```python
from build123d import *

# Parameters (mm, degrees)
F0_R     = 2.4892
F0_R_2   = 2.0193
F0_R_3   = 3.175
F0_R_4   = 1.397
F2_DEPTH = 3
F1_R     = 1.5875
F3_DEPTH = 3.001
F4_W     = 33.02
F4_H     = 15.24
F5_DEPTH = 1.41224


with BuildPart() as f2:
    # F0 (on Top) → F2 (new body)
    with BuildSketch(Plane.XY):
        with BuildLine():
            Line((329.40625, 44.45), (-329.40625, 44.45))
            ThreePointArc((-329.40625, 44.45), (-331.651314, 43.520064), (-332.58125, 41.275))
            Line((-332.58125, 41.275), (-332.58125, -41.275))
            ThreePointArc((-332.58125, -41.275), (-331.651314, -43.520064), (-329.40625, -44.45))
            Line((-329.40625, -44.45), (329.40625, -44.45))
            ThreePointArc((329.40625, -44.45), (331.651314, -43.520064), (332.58125, -41.275))
            Line((332.58125, -41.275), (332.58125, 41.275))
            ThreePointArc((332.58125, 41.275), (331.651314, 43.520064), (329.40625, 44.45))
        make_face()
        with Locations((-326.23125, -38.1)):
            Circle(F0_R, mode=Mode.SUBTRACT)
        with Locations((-121.96875, -35.2)):
            Circle(F0_R_2, mode=Mode.SUBTRACT)
        with Locations((-47.26875, -35.2)):
            Circle(F0_R_2, mode=Mode.SUBTRACT)
        with Locations((-326.23125, -22.225)):
            Circle(F0_R, mode=Mode.SUBTRACT)
        with Locations((-326.23125, -6.35)):
            Circle(F0_R, mode=Mode.SUBTRACT)
        with Locations((27.43125, -35.2)):
            Circle(F0_R_2, mode=Mode.SUBTRACT)
        with Locations((102.13125, -35.2)):
            Circle(F0_R_2, mode=Mode.SUBTRACT)
        with Locations((176.83125, -35.2)):
            Circle(F0_R_2, mode=Mode.SUBTRACT)
        with Locations((251.53125, -35.2)):
            Circle(F0_R_2, mode=Mode.SUBTRACT)
        with Locations((326.23125, -38.1)):
            Circle(F0_R, mode=Mode.SUBTRACT)
        with Locations((326.23125, -22.225)):
            Circle(F0_R, mode=Mode.SUBTRACT)
        with Locations((326.23125, -6.35)):
            Circle(F0_R, mode=Mode.SUBTRACT)
        with Locations((-326.23125, 6.35)):
            Circle(F0_R, mode=Mode.SUBTRACT)
        with Locations((-326.23125, 22.225)):
            Circle(F0_R, mode=Mode.SUBTRACT)
        with Locations((-326.23125, 38.1)):
            Circle(F0_R, mode=Mode.SUBTRACT)
        with Locations((-121.96875, 35.2)):
            Circle(F0_R_2, mode=Mode.SUBTRACT)
        with Locations((-47.26875, 35.2)):
            Circle(F0_R_2, mode=Mode.SUBTRACT)
        with Locations((326.23125, 6.35)):
            Circle(F0_R, mode=Mode.SUBTRACT)
        with Locations((27.43125, 35.2)):
            Circle(F0_R_2, mode=Mode.SUBTRACT)
        with Locations((102.13125, 35.2)):
            Circle(F0_R_2, mode=Mode.SUBTRACT)
        with Locations((326.23125, 22.225)):
            Circle(F0_R, mode=Mode.SUBTRACT)
        with Locations((176.83125, 35.2)):
            Circle(F0_R_2, mode=Mode.SUBTRACT)
        with Locations((251.53125, 35.2)):
            Circle(F0_R_2, mode=Mode.SUBTRACT)
        with Locations((275.43125, 35.2)):
            Circle(F0_R_3, mode=Mode.SUBTRACT)
        with Locations((300.83125, 35.2)):
            Circle(F0_R_4, mode=Mode.SUBTRACT)
        with Locations((326.23125, 38.1)):
            Circle(F0_R, mode=Mode.SUBTRACT)
    extrude(amount=F2_DEPTH)

    # F1 (on face) → F3 (cut, through all)
    with BuildSketch(Plane.XY):
        with BuildLine():
            Line((293.120775, 14.162294), (279.987659, 14.162294))
            ThreePointArc((279.987659, 14.162294), (277.780685, 13.133165), (277.150428, 10.781014))
            Line((277.150428, 10.781014), (277.985866, 6.043014))
            ThreePointArc((277.985866, 6.043014), (278.971226, 4.33632), (280.823097, 3.662294))
            Line((280.823097, 3.662294), (292.285338, 3.662294))
            ThreePointArc((292.285338, 3.662294), (294.137209, 4.33632), (295.122569, 6.043014))
            Line((295.122569, 6.043014), (295.958006, 10.781014))
            ThreePointArc((295.958006, 10.781014), (295.327749, 13.133165), (293.120775, 14.162294))
        make_face()
        with Locations((274.054217, 8.912294)):
            Circle(F1_R)
        with Locations((299.054217, 8.912294)):
            Circle(F1_R)
    extrude(amount=F3_DEPTH, mode=Mode.SUBTRACT)

    # F4 (on face) → F5 (cut)
    with BuildSketch(Plane.XY.offset(3)):
        with Locations((286.554217, 8.912294)):
            Rectangle(F4_W, F4_H)
    extrude(amount=-F5_DEPTH, mode=Mode.SUBTRACT)


solid = f2.part
```
Model file for the job. Use its own axes, mm. Coordinates: 2 decimals unless noted, no trailing zeros. Return JSON: item names as keys, results as strings.
Item 1: Pin check, flat tips, straight feed: P1, Ø5, axis at x = 299.05, y = 8.91, coming from the +Z side; P2, Ø4.5, axis at x = 27.43, y = 35.2, coming from the -Z side. Stop position of each tip, or through.
Model answer:
{"P1": "stops at z = 1.59", "P2": "stops at z = 0"}
Item 2: Wall check: line 1 along X through (y, z) = (21.5, 1.5); line 2 along Y through (x, z) = (276, 2.4); line 3 along Y through (x, z) = (295, 2.4). Give the ranges that are in metal, low to high. Write a range as from..to.
Model answer:
{"line 1": "x = -332.58..-328.61, -323.85..323.85, 328.61..332.58", "line 2": "y = -44.45..1.29, 16.53..32.08, 38.32..44.45", "line 3": "y = -44.45..1.29, 16.53..44.45"}
Item 3: Mould opens along Y. For faces 1 (the face through (286, 2, 1.588)), 2 (the face through (-5, 1, 3)) say: pulls with the +Y half, pulls with the -Y half, needs draft (parallel to the pull), parting line crosses it, or undercut.
Model answer:
{"face 1": "undercut", "face 2": "needs draft"}
